Could you check a few things on this model? Use its own coordinates, in mm. Face numbers are marked on the shaded views. A direction names the side the tool comes from. Coordinates: 2 decimals unless noted, no trailing zeros. Loops run counter-clockwise (first coordinate to the right, second up) from the corner with the lowest first, then second, coordinate; pieces in that order, holes last. Notation, with made-up numbers: M -5,-4 L 54,-4 A31 cw 54,31 Z; hole C -20,84.5 d5. An arc over 180 degrees is marked long. Use one line per item in the form item = value. Start each with the question number.
```python
from build123d import *

# Parameters (mm, degrees)
SKETCH1_W           = 60
SKETCH1_H           = 40
BOSS_EXTRUDE1_DEPTH = 5
SKETCH2_W           = 34.2
SKETCH2_H           = 46
CUT_EXTRUDE1_DEPTH  = 73.284161474
SKETCH3_R           = 1.15
CUT_EXTRUDE2_DEPTH  = 73.284161474
SKETCH4_R           = 2.15
CUT_EXTRUDE3_DEPTH  = 2.4
SKETCH5_W           = 36
SKETCH5_H           = 56.5
CUT_EXTRUDE4_DEPTH  = 1.2
SKETCH6_W           = 25
SKETCH6_H           = 3
CUT_EXTRUDE5_DEPTH  = 2.5
FILLET1_R           = 1
BOSS_EXTRUDE2_REACH = 72.721
SKETCH7_W           = 6.5
SKETCH7_H           = 1.5


with BuildPart() as part:
    # Sketch1 → Boss-Extrude1 (new body)
    with BuildSketch(Plane(origin=(0, 0, 0), x_dir=(0, 1, 0), z_dir=(0, 0, 1))):
        with Locations((30, -20)):
            Rectangle(SKETCH1_W, SKETCH1_H)
    extrude(amount=BOSS_EXTRUDE1_DEPTH)

    # Sketch2 → Cut-Extrude1 (cut, through all)
    with BuildSketch(Plane(origin=(0, 0, 0), x_dir=(1, 0, 0), z_dir=(0, 0, -1))):
        with Locations((20, -30)):
            Rectangle(SKETCH2_W, SKETCH2_H)
    extrude(amount=-CUT_EXTRUDE1_DEPTH, mode=Mode.SUBTRACT)

    # Sketch3 → Cut-Extrude2 (cut, through all)
    with BuildSketch(Plane.XY.offset(5)):
        with Locations((5, 4.5)):
            Circle(SKETCH3_R)
        with Locations((35, 4.5)):
            Circle(SKETCH3_R)
        with Locations((5, 55.5)):
            Circle(SKETCH3_R)
        with Locations((35, 55.5)):
            Circle(SKETCH3_R)
    extrude(amount=-CUT_EXTRUDE2_DEPTH, mode=Mode.SUBTRACT)

    # Sketch4 → Cut-Extrude3 (cut)
    with BuildSketch(Plane.XY.offset(5)):
        with Locations((5, 55.5)):
            Circle(SKETCH4_R)
        with Locations((35, 55.5)):
            Circle(SKETCH4_R)
        with Locations((5, 4.5)):
            Circle(SKETCH4_R)
        with Locations((35, 4.5)):
            Circle(SKETCH4_R)
    extrude(amount=-CUT_EXTRUDE3_DEPTH, mode=Mode.SUBTRACT)

    # Sketch5 → Cut-Extrude4 (cut)
    with BuildSketch(Plane(origin=(0, 0, 0), x_dir=(1, 0, 0), z_dir=(0, 0, -1))):
        with Locations((20, -30)):
            Rectangle(SKETCH5_W, SKETCH5_H)
    extrude(amount=-CUT_EXTRUDE4_DEPTH, mode=Mode.SUBTRACT)

    # Sketch6 → Cut-Extrude5 (cut)
    with BuildSketch(Plane(origin=(0, 0, 1.2), x_dir=(1, 0, 0), z_dir=(0, 0, -1))):
        with Locations((20, -55.625)):
            Rectangle(SKETCH6_W, SKETCH6_H)
    extrude(amount=-CUT_EXTRUDE5_DEPTH, mode=Mode.SUBTRACT)

    # Fillet1
    fillet1_edges = [part.edges().sort_by_distance(p)[0] for p in [
        (20, 60, 5),
        (0, 30, 5),
        (20, 0, 5),
        (40, 30, 5),
    ]]
    fillet(fillet1_edges, radius=FILLET1_R)

    # Sketch7 → Boss-Extrude2 (add, up to next)
    with BuildSketch(Plane.YZ.offset(2.9), mode=Mode.PRIVATE) as boss_extrude2_sk1:
        with Locations((10.25, 4.25)):
            Rectangle(SKETCH7_W, SKETCH7_H)
    boss_extrude2_tool1 = extrude(boss_extrude2_sk1.sketch, amount=BOSS_EXTRUDE2_REACH, mode=Mode.PRIVATE) - part.part
    add(boss_extrude2_tool1.solids().sort_by_distance((2.9, 10.25, 4.25))[0])


solid = part.part
```
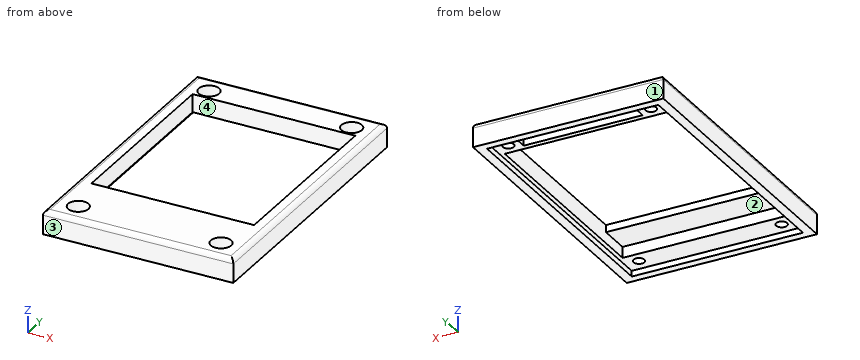
Item 1: I'm going to push flat-ended pins straight in: P1, Ø2.5, axis at x = 5, y = 55.5, coming from the +Z side; P2, Ø2, axis at x = 4.5, y = 18.5, coming from the -Z side; P3, Ø3.5, axis at x = 35, y = 5, coming from the +Z side; P4, Ø3.5, axis at x = 35, y = 4.5, coming from the -Z side. Where does each tip first touch, or does it pass through?
Item 2: I want a section at D-D (x = 12.5). Write out the boundary of the cut face in (y, z) (3 decimals), plus the area to 3 significant figures.
Item 3: For the marked faces 3 and 4, which set-ups out of +Z, -Z, +X, -X, +Y, -Y let a thin tool reach every point of the face, with its end or its side?
Item 4: Thinking about a two-plate mould opening in X: for the marked faces 1 and 2, which applies, pulls with the +X half, pulls with the -X half, needs draft (parallel to the pull), parting line crosses it, or undercut?
Item 5: Please list where these lines run through material, in increasing order: line 1 along Y through (x, z) = (16.5, 2.9) (3 decimals); line 2 along Y through (x, z) = (35, 1.9); line 3 along X through (y, z) = (20.5, 3).
Item 6: I want a section at A-A (x = 35). Count the separate pieces of the cut face and the enclosed holes in it, plus the area to 3 significant figures.
Item 7: I want a section at C-C (y = 40). Write out the boundary of the cut face in (x, z).
Worked answers:
q1.P1 = 2.6
q1.P2 = through
q1.P3 = 5
q1.P4 = 1.2
q2.outline = M 0,0 L 1.75,0 L 1.75,1.2 L 7,1.2 L 7,3.5 L 13.5,3.5 L 13.5,5 L 1,5 A1 ccw 0,4 Z; M 53,1.2 L 54.125,1.2 L 54.125,3.7 L 57.125,3.7 L 57.125,1.2 L 58.25,1.2 L 58.25,0 L 60,0 L 60,4 A1 ccw 59,5 L 53,5 Z
q2.area = 59.2 mm²
q3.face_3 = +Z, -Z, +X, -X, -Y
q3.face_4 = +Z, -Z
q4.face_1 = needs draft
q4.face_2 = undercut
q5.line_1 = 0 to 7, 53 to 54.125, 57.125 to 60
q5.line_2 = 0 to 3.35, 5.65 to 7, 53 to 54.35, 56.65 to 60
q5.line_3 = 0 to 2.9, 37.1 to 40
q6.separate_pieces = 4
q6.enclosed_holes = 0
q6.area = 39.6 mm²
q7.outline = M 0,0 L 2,0 L 2,1.2 L 2.9,1.2 L 2.9,5 L 1,5 A1 ccw 0,4 Z; M 37.1,1.2 L 38,1.2 L 38,0 L 40,0 L 40,4 A1 ccw 39,5 L 37.1,5 Z
